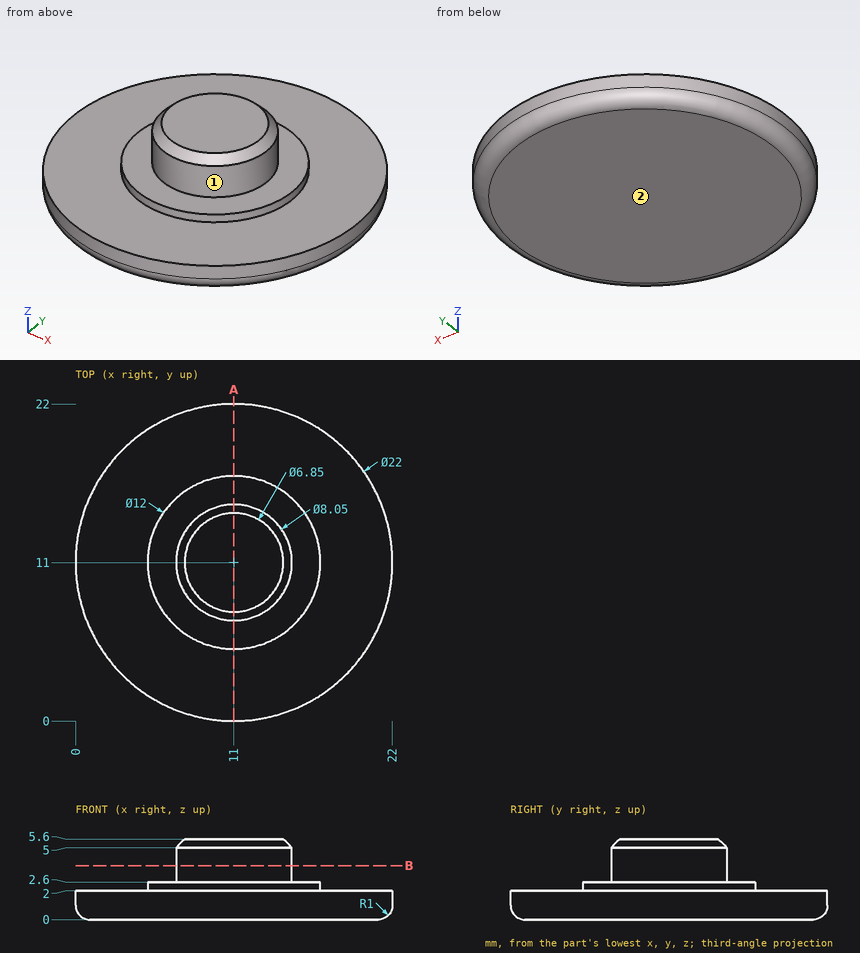
Print and shaded views of the part. All mm, measured from the part's lowest x, y and z. A direction names the side the tool comes from. Round coordinates to 2 decimals unless told otherwise and drop trailing zeros. Order: outer loops, then holes, each group sorted by start corner. A loop starts at its lowest first (then second) coordinate and runs counter-clockwise, first axis right, second up.
Q1. Which spindle directions (+Z, -Z, +X, -X, +Y, -Y) get a long thin tool onto all of the face, cutting with end or side? Do the marked faces 1 and 2. Say none if no direction does.
Q2. Slice it at B-B (z = 3.75). Write the cut outline in (x, y) (3 decimals).
Q3. Drop flat-ended pins along their axis: pin 1 (1.5 mm diameter, centred on x = 4.5, z = 1.5, fed in from -Y); pin 2 (1.5 mm diameter, centred on y = 16.5, z = 1, fed in from -X). Give the stop position or say it passes through.
Q4. Slice it at A-A (x = 11). Write the cut outline in (y, z) (3 decimals), and give its area (3 significant figures).
Q5. Wall check: L1, parallel to Z at x = 17, y = 13.25; L2, parallel to Y at x = 11, z = 2.1; L3, parallel to Z at x = 16.5, y = 12. Give the ranges that are in metal, low to high.
Results below:
1. face 1: +Z
1. face 2: -Z, +X, -X, +Y, -Y
2. outline: circle Ø8.05 at (11, 11)
3. pin 1: stops at y = 1.62
3. pin 2: stops at x = 1.08
4. outline: (0, 1) arc R1 ccw to (1, 0) - (21, 0) arc R1 ccw to (22, 1) - (22, 2) - (17, 2) - (17, 2.6) - (15.025, 2.6) - (15.025, 5) - (14.425, 5.6) - (7.575, 5.6) - (6.975, 5) - (6.975, 2.6) - (5, 2.6) - (5, 2) - (0, 2) - close
4. area: 74.6 mm2
5. L1: z = 0 to 2
5. L2: y = 5 to 17
5. L3: z = 0 to 2.6
